Design review of the part shown in the three views and the two pictorial views. Dimensions are in mm from the part's minimum x, y and z. A direction names the side the tool comes from. Coordinates: 2 decimals unless noted, no trailing zeros. Write each loop counter-clockwise with the first axis right and the second up, starting at its lowest first coordinate (ties: lowest second). Pieces come first, ordered by that corner, then holes. Notation, with made-up numbers: (-10, 9.5) - (26, 9.5) arc R17 cw to (26, 27.5) - close; hole circle Ø2 at (41, -35.75). An arc over 180 degrees is marked (long way). Return JSON: item names as keys, results as strings. Group by question number.
(1) To check wall thickness, follow L1, parallel to X at y = 3.2, z = 2.5; L2, parallel to Z at x = 5, y = 1; L3, parallel to Y at x = 23.5, z = 9.5. State the ranges of each line that lie inside material, in increasing order. Write a range as from..to.
(2) Tool access review of the marked faces 4 and 5: name each direction out of +Z, -Z, +X, -X, +Y, -Y from which nothing blocks a thin tool from reaching the whole face with its end or side.
(3) We need section C-C on x = 13.5. State the section outline as (y, z) points.
(4) We need section B-B on x = 5.5. State the section outline as (y, z) points, then the cut area to 3 significant figures.
(5) For pin 1 Ø1.2 at (x, z) = (11.5, 10.5) entering from -Y; pin 2 Ø1.2 at (x, y) = (6.5, 0.5) entering from +Z, all flat-tipped, find the tip position at first contact; note any pin that passes through.
(6) We need section D-D on y = 2.05. State the section outline as (x, z) points, then the cut area to 3 significant figures.
(7) Draft analysis for pull direction X (two halves, no side actions). For the marked faces 1, 2 and 3, state which applies: released by +X, released by -X, zero draft, split by the parting line, or undercut.
(8) We need section A-A on z = 1.75. State the section outline as (x, y) points.
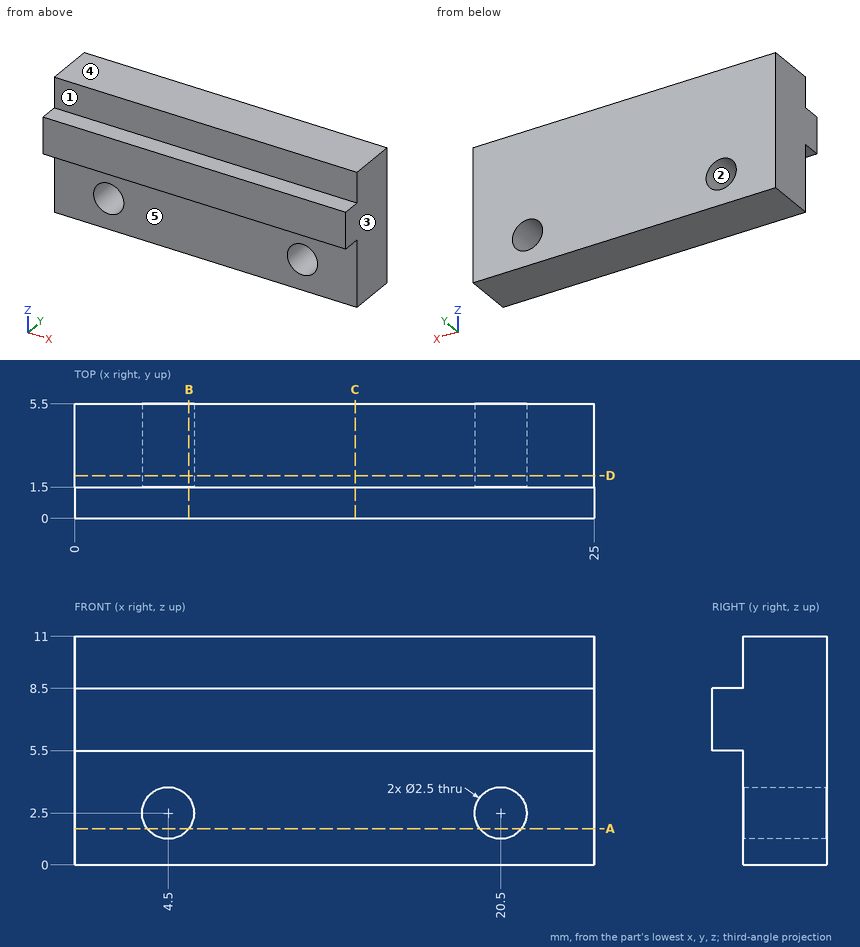
Ans:
{
 "1": {"L1": "0..3.25, 5.75..19.25, 21.75..25", "L2": "5.5..8.5", "L3": "1.5..5.5"},
 "2": {"face 4": "+Z, +X, -X, +Y, -Y", "face 5": "-Z, +X, -X, -Y"},
 "3": {"outline": "(0, 5.5) - (1.5, 5.5) - (1.5, 0) - (5.5, 0) - (5.5, 11) - (1.5, 11) - (1.5, 8.5) - (0, 8.5) - close"},
 "4": {"outline": "(0, 5.5) - (1.5, 5.5) - (1.5, 3.25) - (5.5, 3.25) - (5.5, 11) - (1.5, 11) - (1.5, 8.5) - (0, 8.5) - close; (1.5, 0) - (5.5, 0) - (5.5, 1.75) - (1.5, 1.75) - close", "area": "42.5 mm²"},
 "5": {"pin 1": "y = 1.5", "pin 2": "z = 8.5"},
 "6": {"outline": "(0, 0) - (25, 0) - (25, 11) - (0, 11) - close; hole circle Ø2.5 at (4.5, 2.5); hole circle Ø2.5 at (20.5, 2.5)", "area": "265 mm²"},
 "7": {"face 1": "zero draft", "face 2": "undercut", "face 3": "released by +X"},
 "8": {"outline": "(0, 1.5) - (3.5, 1.5) - (3.5, 5.5) - (0, 5.5) - close; (5.5, 1.5) - (19.5, 1.5) - (19.5, 5.5) - (5.5, 5.5) - close; (21.5, 1.5) - (25, 1.5) - (25, 5.5) - (21.5, 5.5) - close"}
}
